from build123d import *

# Parameters (mm, degrees)
SKETCH1_W           = 290
SKETCH1_H           = 98
SKETCH1_R           = 1.65
SKETCH1_R_2         = 1.7
BOSS_EXTRUDE1_DEPTH = 6


with BuildPart() as part:
    # Sketch1 → Boss-Extrude1 (new body)
    with BuildSketch(Plane(origin=(0, 0, -9.5), x_dir=(-1, 0, 0), z_dir=(0, 0, -1))):
        with Locations((127, 40)):
            Rectangle(SKETCH1_W, SKETCH1_H)
        with Locations(Location((264, 0, 0), (0, 0, 180))):
            Circle(SKETCH1_R, mode=Mode.SUBTRACT)
        with Locations(Location((248, 0, 0), (0, 0, 180))):
            Circle(SKETCH1_R, mode=Mode.SUBTRACT)
        with Locations(Location((248, 10, 0), (0, 0, 180))):
            Circle(SKETCH1_R, mode=Mode.SUBTRACT)
        with Locations(Location((264, 10, 0), (0, 0, 180))):
            Circle(SKETCH1_R, mode=Mode.SUBTRACT)
        with Locations(Location((248, 45.003288428, 0), (0, 0, 180))):
            Circle(SKETCH1_R, mode=Mode.SUBTRACT)
        with Locations(Location((264, 35.003288428, 0), (0, 0, 180))):
            Circle(SKETCH1_R, mode=Mode.SUBTRACT)
        with Locations(Location((248, 80, 0), (0, 0, 180))):
            Circle(SKETCH1_R, mode=Mode.SUBTRACT)
        with Locations(Location((264, 70, 0), (0, 0, 180))):
            Circle(SKETCH1_R, mode=Mode.SUBTRACT)
        with Locations(Location((24, 0, 0), (0, 0, 180))):
            Circle(SKETCH1_R_2, mode=Mode.SUBTRACT)
        with Locations(Location((236, 0, 0), (0, 0, 180))):
            Circle(SKETCH1_R_2, mode=Mode.SUBTRACT)
        with Locations(Location((248, 70, 0), (0, 0, 180))):
            Circle(SKETCH1_R, mode=Mode.SUBTRACT)
        with Locations(Location((264, 80, 0), (0, 0, 180))):
            Circle(SKETCH1_R, mode=Mode.SUBTRACT)
        with Locations(Location((248, 35.003288428, 0), (0, 0, 180))):
            Circle(SKETCH1_R, mode=Mode.SUBTRACT)
        with Locations(Location((264, 45.003288428, 0), (0, 0, 180))):
            Circle(SKETCH1_R, mode=Mode.SUBTRACT)
        with BuildLine():
            Line((-11, 71.65), (15, 71.65))
            ThreePointArc((15, 71.65), (16.65, 70), (15, 68.35))
            Line((15, 68.35), (-11, 68.35))
            ThreePointArc((-11, 68.35), (-12.65, 70), (-11, 71.65))
        make_face(mode=Mode.SUBTRACT)
        with BuildLine():
            Line((-11, 81.65), (15, 81.65))
            ThreePointArc((15, 81.65), (16.65, 80), (15, 78.35))
            Line((15, 78.35), (-11, 78.35))
            ThreePointArc((-11, 78.35), (-12.65, 80), (-11, 81.65))
        make_face(mode=Mode.SUBTRACT)
        with BuildLine():
            Line((15, -1.65), (-11, -1.65))
            ThreePointArc((-11, -1.65), (-12.65, 0), (-11, 1.65))
            Line((-11, 1.65), (15, 1.65))
            ThreePointArc((15, 1.65), (16.65, 0), (15, -1.65))
        make_face(mode=Mode.SUBTRACT)
        with BuildLine():
            Line((15, 8.35), (-11, 8.35))
            ThreePointArc((-11, 8.35), (-12.65, 10), (-11, 11.65))
            Line((-11, 11.65), (15, 11.65))
            ThreePointArc((15, 11.65), (16.65, 10), (15, 8.35))
        make_face(mode=Mode.SUBTRACT)
        with BuildLine():
            Line((124, -1.7), (44, -1.7))
            ThreePointArc((44, -1.7), (42.3, 0), (44, 1.7))
            Line((44, 1.7), (124, 1.7))
            ThreePointArc((124, 1.7), (125.7, 0), (124, -1.7))
        make_face(mode=Mode.SUBTRACT)
        with BuildLine():
            Line((25.7, 80), (25.7, 20))
            ThreePointArc((25.7, 20), (24, 18.3), (22.3, 20))
            Line((22.3, 20), (22.3, 80))
            ThreePointArc((22.3, 80), (24, 81.7), (25.7, 80))
        make_face(mode=Mode.SUBTRACT)
        with BuildLine():
            Line((216, -1.7), (136, -1.7))
            ThreePointArc((136, -1.7), (134.3, 0), (136, 1.7))
            Line((136, 1.7), (216, 1.7))
            ThreePointArc((216, 1.7), (217.7, 0), (216, -1.7))
        make_face(mode=Mode.SUBTRACT)
        with BuildLine():
            Line((237.7, 80), (237.7, 20))
            ThreePointArc((237.7, 20), (236, 18.3), (234.3, 20))
            Line((234.3, 20), (234.3, 80))
            ThreePointArc((234.3, 80), (236, 81.7), (237.7, 80))
        make_face(mode=Mode.SUBTRACT)
        with BuildLine():
            Line((15, 33.346711572), (-11, 33.346711572))
            ThreePointArc((-11, 33.346711572), (-12.65, 34.996711572), (-11, 36.646711572))
            Line((-11, 36.646711572), (15, 36.646711572))
            ThreePointArc((15, 36.646711572), (16.65, 34.996711572), (15, 33.346711572))
        make_face(mode=Mode.SUBTRACT)
        with BuildLine():
            Line((15, 43.346711572), (-11, 43.346711572))
            ThreePointArc((-11, 43.346711572), (-12.65, 44.996711572), (-11, 46.646711572))
            Line((-11, 46.646711572), (15, 46.646711572))
            ThreePointArc((15, 46.646711572), (16.65, 44.996711572), (15, 43.346711572))
        make_face(mode=Mode.SUBTRACT)
    extrude(amount=-BOSS_EXTRUDE1_DEPTH)


solid = part.part
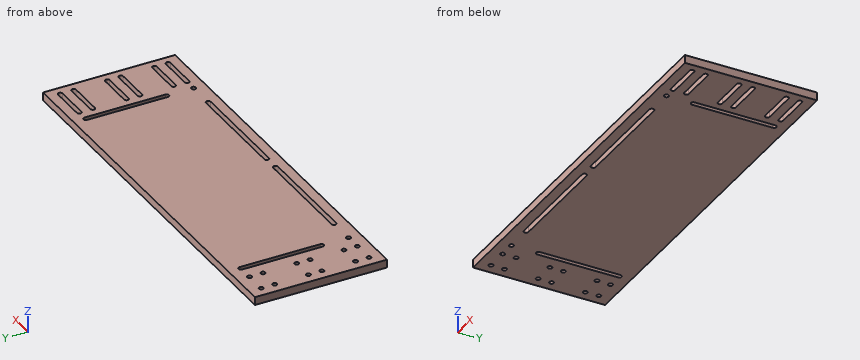
Work out the finished part from the listing and answer in its coordinate system (mm). Give positions to 0.01 mm unless a question says otherwise; leave off trailing zeros. Order: outer loops, then holes, each group sorted by start corner. A loop starts at its lowest first (then second) coordinate and runs counter-clockwise, first axis right, second up. Notation, with made-up numbers: (30.25, 28) -> (47.25, 28) arc R26 cw to (47.25, 46) -> close; hole circle Ø6 at (68, 76). An arc over 180 degrees is marked (long way). Answer as a JSON object with one key per item and string values. Group by question number.
1. A flat-ended cylindrical pin translates along its axis: pin 1 Ø3 at (x, y) = (-264, 70) entering from -Z. Find the tip coordinate at first contact, or state that the pin passes through.
2. Section B-B on x = -184.5 is taken. Determine the outline of the cut face in (y, z).
3. Section A-A on y = 56 is taken. Determine the outline of the cut face in (x, z).
4. Section C-C on z = -5.7 is taken. Count the separate pieces of the cut face and the enclosed holes in it, plus the area to 3 significant figures.
5. Consider line 1 along X through (y, z) = (40.5, -3.9); line 2 along X through (y, z) = (10, -5); line 3 along Y through (x, z) = (-179, -8.45). Determine where each line is inside the solid, lowest interval first. Write a range as [from, to].
Result sheet:
{
 "1": {"pin 1": "passes through"},
 "2": {"outline": "(-9, -9.5) -> (-1.7, -9.5) -> (-1.7, -3.5) -> (-9, -3.5) -> close; (1.7, -9.5) -> (89, -9.5) -> (89, -3.5) -> (1.7, -3.5) -> close"},
 "3": {"outline": "(-272, -9.5) -> (-237.7, -9.5) -> (-237.7, -3.5) -> (-272, -3.5) -> close; (-234.3, -9.5) -> (-25.7, -9.5) -> (-25.7, -3.5) -> (-234.3, -3.5) -> close; (-22.3, -9.5) -> (18, -9.5) -> (18, -3.5) -> (-22.3, -3.5) -> close"},
 "4": {"separate pieces": "1", "enclosed holes": "24", "area": "26,700 mm^2"},
 "5": {"line 1": "x = [-272, -237.7], [-234.3, -25.7], [-22.3, 18]", "line 2": "x = [-272, -265.65], [-262.35, -249.65], [-246.35, -16.65], [12.65, 18]", "line 3": "y = [-9, -1.7], [1.7, 89]"}
}
